from build123d import *

# Parameters (mm, degrees)
F1_DEPTH = 3


# Not quite as in the source:
# - ends of sketch curves that miss each other by under 0.0002 mm in the source are joined


with BuildPart() as f1:
    # F0 (on Front) → F1 (new body)
    with BuildSketch(Plane.XZ):
        with BuildLine():
            Line((60.097833329, -50), (73.431166662, -50))
            Line((73.431166662, -50), (73.431166662, -47))
            Line((73.431166662, -47), (86.7645, -47))
            Line((86.7645, -47), (86.7645, -50.0000007451))
            Line((86.7645, -50.0000007451), (100.097833333, -50.0000007451))
            Line((100.097833333, -50.0000007451), (100.097833333, -47.0000007451))
            Line((100.097833333, -47.0000007451), (113.2355, -47.0000007451))
            Line((113.2355, -47.0000007451), (113.2355, -35.714285716))
            Line((113.2355, -35.714285716), (110.2355, -35.714285716))
            Line((110.2355, -35.714285716), (110.2355, -21.42857143))
            Line((110.2355, -21.42857143), (113.2355, -21.42857143))
            Line((113.2355, -21.42857143), (113.2355, -7.142857144))
            Line((113.2355, -7.142857144), (110.2355, -7.142857144))
            Line((110.2355, -7.142857144), (110.2355, 7.142857142))
            Line((110.2355, 7.142857142), (113.2355, 7.142857142))
            Line((113.2355, 7.142857142), (113.2355, 21.428571428))
            Line((113.2355, 21.428571428), (110.2355, 21.428571428))
            Line((110.2355, 21.428571428), (110.2355, 35.714285714))
            Line((110.2355, 35.714285714), (113.2355, 35.714285714))
            Line((113.2355, 35.714285714), (113.2355, 50))
            Line((113.2355, 50), (93.2355, 50))
            Line((93.2355, 50), (71.8119617716, -22.2537644208))
            ThreePointArc((71.8119617716, -22.2537644208), (68.2066991862, -27.4243868361), (62.2245235205, -29.4110495597))
            Line((62.2245235205, -29.4110495597), (0, -29.4110495597))
            Line((0, -29.4110495597), (-62.2245235205, -29.4110495597))
            ThreePointArc((-62.2245235205, -29.4110495597), (-68.2066991862, -27.4243868361), (-71.8119617716, -22.2537644208))
            Line((-71.8119617716, -22.2537644208), (-93.2355, 50))
            Line((-93.2355, 50), (-113.2355, 50))
            Line((-113.2355, 50), (-113.2355, 35.714285714))
            Line((-113.2355, 35.714285714), (-110.2355, 35.714285714))
            Line((-110.2355, 35.714285714), (-110.2355, 21.428571428))
            Line((-110.2355, 21.428571428), (-113.2355, 21.428571428))
            Line((-113.2355, 21.428571428), (-113.2355, 7.142857142))
            Line((-113.2355, 7.142857142), (-110.2355, 7.142857142))
            Line((-110.2355, 7.142857142), (-110.2355, -7.142857144))
            Line((-110.2355, -7.142857144), (-113.2355, -7.142857144))
            Line((-113.2355, -7.142857144), (-113.2355, -21.42857143))
            Line((-113.2355, -21.42857143), (-110.2355, -21.42857143))
            Line((-110.2355, -21.42857143), (-110.2355, -35.714285716))
            Line((-110.2355, -35.714285716), (-113.2355, -35.714285716))
            Line((-113.2355, -35.714285716), (-113.2355, -47))
            Line((-113.2355, -47), (-99.902166667, -47))
            Line((-99.902166667, -47), (-99.902166667, -50))
            Line((-99.902166667, -50), (-86.568833334, -50))
            Line((-86.568833334, -50), (-86.568833334, -47))
            Line((-86.568833334, -47), (-73.235500001, -47))
            Line((-73.235500001, -47), (-73.235500001, -50))
            Line((-73.235500001, -50), (-59.902166668, -50))
            Line((-59.902166668, -50), (-59.902166668, -47))
            Line((-59.902166668, -47), (-46.568833335, -47))
            Line((-46.568833335, -47), (-46.568833335, -50))
            Line((-46.568833335, -50), (-33.235500002, -50))
            Line((-33.235500002, -50), (-33.235500002, -47))
            Line((-33.235500002, -47), (-19.902166669, -47))
            Line((-19.902166669, -47), (-19.902166669, -50))
            Line((-19.902166669, -50), (-6.568833336, -50))
            Line((-6.568833336, -50), (-6.568833336, -47))
            Line((-6.568833336, -47), (6.764499997, -47))
            Line((6.764499997, -47), (6.764499997, -50))
            Line((6.764499997, -50), (20.09783333, -50))
            Line((20.09783333, -50), (20.09783333, -47))
            Line((20.09783333, -47), (33.431166663, -47))
            Line((33.431166663, -47), (33.431166663, -50))
            Line((33.431166663, -50), (46.764499996, -50))
            Line((46.764499996, -50), (46.764499996, -47))
            Line((46.764499996, -47), (60.097833329, -47))
            Line((60.097833329, -47), (60.097833329, -50))
        make_face()
    extrude(amount=F1_DEPTH)


solid = f1.part
Geometry: final body of the model. Coordinates: model frame, mm. A direction names the side the tool comes from. Round coordinates to 2 decimals unless told otherwise and drop trailing zeros. Order: outer loops, then holes, each group sorted by start corner. A loop starts at its lowest first (then second) coordinate and runs counter-clockwise, first axis right, second up.
Q1. Section C-C, the plane x = 57. Output: boundary loops of the cut face in (y, z).
Result sheet:
outline: (-3, -47) - (0, -47) - (0, -29.41) - (-3, -29.41) - close
Q2. Section B-B, the plane z = 41. Output: boundary loops of the cut face in (x, y).
Result sheet:
outline: (-113.24, -3) - (-90.57, -3) - (-90.57, 0) - (-113.24, 0) - close; (90.57, -3) - (113.24, -3) - (113.24, 0) - (90.57, 0) - close
Q3. Material intervals for probe 1 along Z at (x, y) = (-24, -1); probe 2 along Z at (x, y) = (60.5, -0.5); probe 3 along X at (y, z) = (-2.5, 29.5), sorted ascending.
Result sheet:
probe 1: z = -47 to -29.41
probe 2: z = -50 to -29.41
probe 3: x = -110.24 to -87.16, 87.16 to 110.24
Q4. Section A-A, the plane z = -12.5. Output: boundary loops of the cut face in (x, y), and give its area (3 significant figures).
Result sheet:
outline: (-113.24, -3) - (-74.7, -3) - (-74.7, 0) - (-113.24, 0) - close; (74.7, -3) - (113.24, -3) - (113.24, 0) - (74.7, 0) - close
area: 231 mm2
Q5. Pin query (flat end, axial travel): pin 1 (0.9 mm diameter, centred on x = -112.5, y = -1.5, fed in from -Z); pin 2 (0.9 mm diameter, centred on x = -17, y = -1, fed in from +Z); pin 3 (1.5 mm diameter, centred on y = -1, z = -31, fed in from +X). Return the tip coordinate at first contact, or that it passes through.
Result sheet:
pin 1: stops at z = -47
pin 2: stops at z = -29.41
pin 3: stops at x = 110.24
Q6. Section D-D, the plane z = -33.5. Output: boundary loops of the cut face in (x, y), and give its area (3 significant figures).
Result sheet:
outline: (-110.24, -3) - (110.24, -3) - (110.24, 0) - (-110.24, 0) - close
area: 661 mm2
Q7. Mould query, pull axis X, two halves, no side actions, for faces 3 (the face through (-2, 0, -33)), 4 (the face through (68.28, -1.48, -27.37)). Classes: released by +X, released by -X, zero draft, split by the parting line, or undercut.
Result sheet:
face 3: zero draft
face 4: undercut
Q8. Access query for faces 1 (the face through (-68.13, -1.48, -27.48)), 2 (the face through (-2, -3, -33)). Directions: +Z, -Z, +X, -X, +Y, -Y. A direction counts if a zero-diameter tool reaches every point of the face in a straight line with its end or side. Return the directions, or none.
Result sheet:
face 1: +Z, +Y, -Y
face 2: +Z, -Z, +X, -X, -Y
